Model file for the job. Use its own axes, mm. A direction names the side the tool comes from. Give positions to 0.01 mm unless a question says otherwise; leave off trailing zeros. Loops run counter-clockwise (first coordinate to the right, second up) from the corner with the lowest first, then second, coordinate; pieces in that order, holes last. Notation, with made-up numbers: (16, 88) -> (41, 88) arc R15 ccw to (41, 99) -> close; hole circle Ø5 at (41.5, 82). An arc over 180 degrees is marked (long way). Use CSV: the item, a comma, the result in double quotes. Start each with the question number.
(1) Flat gauge pins, fed straight in: pin 1 (0.8 mm diameter, centred on x = -96, z = 2.5, fed in from +Y); pin 2 (0.5 mm diameter, centred on y = 185.5, z = 2.5, fed in from -X); pin 3 (3 mm diameter, centred on x = -123.825, y = 0, fed in from +Z) (3 decimals); pin 4 (0.5 mm diameter, centred on x = 15, z = 2.5, fed in from -Y). Where does each tip first touch, or does it go through?
(2) Cut at B-B on x = 83. Write the cut outline in (y, z) (1 decimal).
(3) Pull direction X, two halves, no side cores. Call faces 3 (the cylindrical face through (127, 0, 2)), 4 (the cylindrical face through (0.123, 250.823, 2.37)), 5 (the flat face through (-1, 106, 3.175)): pulls with the +X half, pulls with the -X half, needs draft (parallel to the pull), parting line crosses it, or undercut.
(4) Drill centre lines: probe 1 along X at (y, z) = (146.05, 1.6) (3 decimals); probe 2 along X at (y, z) = (11.5, 0.35) (3 decimals); probe 3 along Y at (x, z) = (-98.5, 2.05). Where is each one in solid material? Low to high.
(5) 3-axis set-ups, long thin cutter, end or side, ignore diameter. For faces 1 (the cylindrical face through (-127, 0, 2)), 2 (the flat face through (-1, 59, 0)): which of +Z, -Z, +X, -X, +Y, -Y reach the whole face in a straight line?
(6) Cut at A-A on z = 2.4. State how many separate pieces and enclosed holes the cut face has, then the cut area to 3 significant figures.
from build123d import *

# Parameters (mm, degrees)
F0_R     = 1.2192
F1_DEPTH = 1.5875
F2_R     = 3.17499
F3_R     = 1.2192
F4_DEPTH = 1.5875


# Not quite as in the source:
# - a fillet or chamfer is up to 0.001 mm smaller than in the source, because OpenCascade refuses the exact size


with BuildPart() as f1:
    # F0 (on Top) → F1 (new body)
    with BuildSketch(Plane.XY):
        Polygon((-127, 3.175), (-127, -3.175), (127, -3.175), (127, 3.175), (3.175, 3.175), (3.175, 250.825), (-3.175, 250.825), (-3.175, 3.175), align=None)
        with Locations((-123.825, 0)):
            Circle(F0_R, mode=Mode.SUBTRACT)
        with Locations((-53.5178, 0)):
            Circle(F0_R, mode=Mode.SUBTRACT)
        with Locations((53.5178, 0)):
            Circle(F0_R, mode=Mode.SUBTRACT)
        with Locations((123.825, 0)):
            Circle(F0_R, mode=Mode.SUBTRACT)
        with Locations((0, 146.05)):
            Circle(F0_R, mode=Mode.SUBTRACT)
        with Locations((0, 247.65)):
            Circle(F0_R, mode=Mode.SUBTRACT)
    extrude(amount=F1_DEPTH)

    # F2 (radius 3.175 in the source; OpenCascade refuses exactly that, so slightly less here)
    f2_edges = [f1.edges().sort_by_distance(p)[0] for p in [
        (-127, -3.175, 0.79375),
        (-127, 3.175, 0.79375),
        (127, 3.175, 0.79375),
        (127, -3.175, 0.79375),
        (-3.175, 250.825, 0.79375),
        (3.175, 250.825, 0.79375),
    ]]
    fillet(f2_edges, radius=F2_R)

    # F3 (on face) → F4 (join)
    with BuildSketch(Plane.XY.offset(1.5875)):
        with BuildLine():
            Line((-56.4611037746, 1.190625), (-120.8816962254, 1.190625))
            ThreePointArc((-120.8816962254, 1.190625), (-127, 0), (-120.8816962254, -1.190625))
            Line((-120.8816962254, -1.190625), (-56.4611037746, -1.190625))
            ThreePointArc((-56.4611037746, -1.190625), (-53.5178, -3.175), (-50.5744962254, -1.190625))
            Line((-50.5744962254, -1.190625), (50.5744962254, -1.190625))
            ThreePointArc((50.5744962254, -1.190625), (53.5178, -3.175), (56.4611037746, -1.190625))
            Line((56.4611037746, -1.190625), (120.8816962254, -1.190625))
            ThreePointArc((120.8816962254, -1.190625), (127, 0), (120.8816962254, 1.190625))
            Line((120.8816962254, 1.190625), (56.4611037746, 1.190625))
            ThreePointArc((56.4611037746, 1.190625), (53.5178, 3.175), (50.5744962254, 1.190625))
            Line((50.5744962254, 1.190625), (1.190625, 1.190625))
            Line((1.190625, 1.190625), (1.190625, 143.1066962254))
            ThreePointArc((1.190625, 143.1066962254), (3.175, 146.05), (1.190625, 148.9933037746))
            Line((1.190625, 148.9933037746), (1.190625, 244.7066962254))
            ThreePointArc((1.190625, 244.7066962254), (0, 250.825), (-1.190625, 244.7066962254))
            Line((-1.190625, 244.7066962254), (-1.190625, 148.9933037746))
            ThreePointArc((-1.190625, 148.9933037746), (-3.175, 146.05), (-1.190625, 143.1066962254))
            Line((-1.190625, 143.1066962254), (-1.190625, 1.190625))
            Line((-1.190625, 1.190625), (-50.5744962254, 1.190625))
            ThreePointArc((-50.5744962254, 1.190625), (-53.5178, 3.175), (-56.4611037746, 1.190625))
        make_face()
        with Locations((-123.825, 0)):
            Circle(F3_R, mode=Mode.SUBTRACT)
        with Locations((-53.5178, 0)):
            Circle(F3_R, mode=Mode.SUBTRACT)
        with Locations((53.5178, 0)):
            Circle(F3_R, mode=Mode.SUBTRACT)
        with Locations((123.825, 0)):
            Circle(F3_R, mode=Mode.SUBTRACT)
        with Locations((0, 146.05)):
            Circle(F3_R, mode=Mode.SUBTRACT)
        with Locations((0, 247.65)):
            Circle(F3_R, mode=Mode.SUBTRACT)
    extrude(amount=F4_DEPTH)


solid = f1.part
Check result:
1,pin 1,"y = 1.19"
1,pin 2,"x = -1.19"
1,pin 3,"z = 3.175"
1,pin 4,"y = -1.19"
2,outline,"(-3.2, 0) -> (3.2, 0) -> (3.2, 1.6) -> (1.2, 1.6) -> (1.2, 3.2) -> (-1.2, 3.2) -> (-1.2, 1.6) -> (-3.2, 1.6) -> close"
3,face 3,"undercut"
3,face 4,"parting line crosses it"
3,face 5,"needs draft"
4,probe 1,"-3.175 to -1.219, 1.219 to 3.175"
4,probe 2,"-3.175 to 3.175"
4,probe 3,"-1.19 to 1.19"
5,face 1,"+Z"
5,face 2,"-Z, +X, -X, +Y, -Y"
6,separate pieces,"1"
6,enclosed holes,"6"
6,area,"1,270 mm²"
